Here's how the part is built. I have some questions about the finished solid (model axes, mm). A direction names the side the tool comes from. Give positions to 0.01 mm unless a question says otherwise; leave off trailing zeros. Loops run counter-clockwise (first coordinate to the right, second up) from the corner with the lowest first, then second, coordinate; pieces in that order, holes last. Notation, with made-up numbers: (67.5, 89.25) -> (123.5, 89.25) arc R27 ccw to (123.5, 106.25) -> close; hole circle Ø5 at (89, 24). An arc over 180 degrees is marked (long way). Answer in a Markdown table with one row per item. Add a question column.
Item 1: We'd pull the mould along Z, two halves only. Please class faces 1 (the face through (-3, 12.8, 2)), 2 (the face through (-9.24, 1.41, 3.52)): released by +Z, released by -Z, zero draft, split by the parting line, or undercut.
Item 2: If we section it at A-A (x = -12): Write out the boundary of the cut face in (y, z), then the cut area to 3 significant figures.
Item 3: If I drill on line 1 (X direction, y = 0.25, z = 0.5); line 2 (Y direction, x = -1, z = 2.5); line 3 (X direction, y = -8, z = 1.05), over which ranges is the centre line in solid material (lowest first)?
Item 4: For P1, Ø1, axis at x = -13.5, z = 4, coming from the +Y side; P2, Ø1, axis at x = 7, z = 1.5, coming from the -Y side, each with a flat end and sliding along its axis, tell me the tip position at first contact or that it passes through.
Item 5: If we section it at C-C (x = 9.5): Write out the boundary of the cut face in (y, z), then the cut area to 3 significant figures.
Item 6: If we section it at B-B (z = 4.2): Write out the boundary of the cut face in (x, y).
Item 7: Which directions (+Z, -Z, +X, -X, +Y, -Y) give clear straight access to the entire face, cutting with the end or side of a thin tool? Please do faces 3 (the face through (-9.24, -11.99, 2.46)), 4 (the face through (2.94, 1.35, 3.52)).
```python
from build123d import *

# Parameters (mm, degrees)
ESQUISSE1_W                       = 34
ESQUISSE1_H                       = 25.6
ESQUISSE1_R                       = 1.7
ESQUISSE1_R_2                     = 2.6
BOSS_EXTRU_1_DEPTH                = 5
ENL_V_MAT_EXTRU_2_DEPTH           = 3
ENL_V_MAT_EXTRU_2_DRAFT           = -5
ENL_V_MAT_EXTRU_2_PROFILE_2_DEPTH = 3
ENL_V_MAT_EXTRU_2_PROFILE_2_DRAFT = -5
ENL_V_MAT_EXTRU_3_DEPTH           = 10
CONG_1_R                          = 4


with BuildPart() as part:
    # Esquisse1 → Boss.-Extru.1 (new body)
    with BuildSketch(Plane.XY):
        with Locations((-3.241443597, 0)):
            Rectangle(ESQUISSE1_W, ESQUISSE1_H)
        with Locations((-11.726724972, 0)):
            Circle(ESQUISSE1_R, mode=Mode.SUBTRACT)
        with Locations((-3.241443597, 8.485281374)):
            Circle(ESQUISSE1_R_2, mode=Mode.SUBTRACT)
        with Locations(Location((-3.241443597, -8.485281374, 0), (0, 0, 180))):
            Circle(ESQUISSE1_R_2, mode=Mode.SUBTRACT)
        with Locations(Location((5.243837777, 0, 0), (0, 0, 180))):
            Circle(ESQUISSE1_R, mode=Mode.SUBTRACT)
    extrude(amount=BOSS_EXTRU_1_DEPTH)


with BuildPart() as enl_v_mat_extru_2_tool:
    # Esquisse3 → Enlèv. mat.-Extru.2 (with draft: the straight prism first)
    with BuildSketch(Plane.XY.offset(5)):
        Polygon((-8.278451106, 0), (-10.002588039, 2.986292767), (-13.450861905, 2.986292767), (-15.174998837, 0), (-13.450861905, -2.986292767), (-10.002588039, -2.986292767), align=None)
    extrude(amount=-ENL_V_MAT_EXTRU_2_DEPTH)
    # Enlèv. mat.-Extru.2: the draft: its side faces are tilted about the plane it starts from
    enl_v_mat_extru_2_sides = [enl_v_mat_extru_2_tool.faces().sort_by_distance(p)[0] for p in [
        (-9.140519572, 1.493146384, 3.5),
        (-11.726724972, 2.986292767, 3.5),
        (-14.312930371, 1.493146384, 3.5),
        (-14.312930371, -1.493146384, 3.5),
        (-11.726724972, -2.986292767, 3.5),
        (-9.140519572, -1.493146384, 3.5),
    ]]
    draft(enl_v_mat_extru_2_sides, Plane.XY.offset(5), ENL_V_MAT_EXTRU_2_DRAFT)


with BuildPart() as part_1:
    add(part.part)

    # Enlèv. mat.-Extru.2: cut by enl_v_mat_extru_2_tool
    add(enl_v_mat_extru_2_tool.part, mode=Mode.SUBTRACT)


with BuildPart() as enl_v_mat_extru_2_profile_2_tool:
    # Esquisse3 → Enlèv. mat.-Extru.2 profile 2 (with draft: the straight prism first)
    with BuildSketch(Plane.XY.offset(5)):
        Polygon((8.476999284, 0), (6.860418531, 2.8), (3.627257023, 2.8), (2.010676269, 0), (3.627257023, -2.8), (6.860418531, -2.8), align=None)
    extrude(amount=-ENL_V_MAT_EXTRU_2_PROFILE_2_DEPTH)
    # Enlèv. mat.-Extru.2 profile 2: the draft: its side faces are tilted about the plane it starts from
    enl_v_mat_extru_2_profile_2_sides = [enl_v_mat_extru_2_profile_2_tool.faces().sort_by_distance(p)[0] for p in [
        (7.668708907, 1.4, 3.5),
        (5.243837777, 2.8, 3.5),
        (2.818966646, 1.4, 3.5),
        (2.818966646, -1.4, 3.5),
        (5.243837777, -2.8, 3.5),
        (7.668708907, -1.4, 3.5),
    ]]
    draft(enl_v_mat_extru_2_profile_2_sides, Plane.XY.offset(5), ENL_V_MAT_EXTRU_2_PROFILE_2_DRAFT)


with BuildPart() as part_2:
    add(part_1.part)

    # Enlèv. mat.-Extru.2 profile 2: cut by enl_v_mat_extru_2_profile_2_tool
    add(enl_v_mat_extru_2_profile_2_tool.part, mode=Mode.SUBTRACT)

    # Esquisse4 → Enlèv. mat.-Extru.3 (cut)
    with BuildSketch(Plane(origin=(0, 0, 0), x_dir=(-1, 0, 0), z_dir=(0, 0, -1))):
        with BuildLine():
            Line((10.241443597, 12.8), (20.241443597, 12.8))
            Line((20.241443597, 12.8), (20.241443597, 2.8))
            ThreePointArc((20.241443597, 2.8), (13.170375785, 5.728932188), (10.241443597, 12.8))
        make_face()
        with BuildLine():
            Line((20.241443597, -12.8), (20.241443597, -2.8))
            ThreePointArc((20.241443597, -2.8), (13.170375785, -5.728932188), (10.241443597, -12.8))
            Line((10.241443597, -12.8), (20.241443597, -12.8))
        make_face()
        with BuildLine():
            Line((-3.758556403, -12.8), (-13.758556403, -12.8))
            Line((-13.758556403, -12.8), (-13.758556403, -2.8))
            ThreePointArc((-13.758556403, -2.8), (-6.687488591, -5.728932188), (-3.758556403, -12.8))
        make_face()
        with BuildLine():
            Line((-13.758556403, 12.8), (-13.758556403, 2.8))
            ThreePointArc((-13.758556403, 2.8), (-6.687488591, 5.728932188), (-3.758556403, 12.8))
            Line((-3.758556403, 12.8), (-13.758556403, 12.8))
        make_face()
    extrude(amount=-ENL_V_MAT_EXTRU_3_DEPTH, mode=Mode.SUBTRACT)

    # Congé1
    # the kernel refuses this fillet: 4 mm, written as the material it takes off along each edge
    with BuildSketch(Plane(origin=(-10.241443597, -12.8, -8.541019662), x_dir=(1, 0, 0), z_dir=(0, 0, 1)), Plane(origin=(-20.241443597, 2.8, -8.541019662), x_dir=(0, -1, 0), z_dir=(0, 0, 1)), Plane(origin=(3.758556403, 12.8, -8.541019662), x_dir=(-1, 0, 0), z_dir=(0, 0, 1))) as cong_1_piece_1:
        with BuildLine():
            CenterArc((3.416407865, 4), CONG_1_R, 196.601549599, 73.398450401)
            ThreePointArc((-0.416851525, 2.857142857), (-0.104761631, 1.443695821), (0, 0))
            Line((0, 0), (3.416407865, 0))
        make_face()
    extrude(amount=22.082039325, mode=Mode.SUBTRACT)
    with BuildSketch(Plane(origin=(-20.241443597, -2.8, -8.541019662), x_dir=(0.9895238368781002, -0.14436958214957515, 0), z_dir=(0, 0, 1)), Plane(origin=(-10.241443597, 12.8, -8.541019662), x_dir=(-0.14436958214957388, -0.9895238368781005, 0), z_dir=(0, 0, 1)), Plane(origin=(13.758556403, 2.8, -8.541019662), x_dir=(-0.9895238368781005, 0.14436958214957332, 0), z_dir=(0, 0, 1))) as cong_1_piece_2:
        with BuildLine():
            CenterArc((3.464869972, 3.958095348), CONG_1_R, 188.300774799, 73.398450401)
            Line((-0.493225376, 3.380617019), (0, 0))
            ThreePointArc((0, 0), (1.443695821, 0.104761631), (2.887391643, 0))
        make_face()
    extrude(amount=22.082039325, mode=Mode.SUBTRACT)
    with BuildSketch(Plane(origin=(3.758556403, -12.8, -8.541019662), x_dir=(-1, 0, 0), z_dir=(0, 0, 1))) as cong_1_piece_3:
        with BuildLine():
            CenterArc((3.416407865, -4), CONG_1_R, 90, 73.398450401)
            ThreePointArc((-0.416851525, -2.857142857), (-0.104761631, -1.443695821), (0, 0))
            Line((0, 0), (3.416407865, 0))
        make_face()
    extrude(amount=22.082039325, mode=Mode.SUBTRACT)
    with BuildSketch(Plane(origin=(13.758556403, -2.8, -8.541019662), x_dir=(-0.9895238368781001, -0.14436958214957546, 0), z_dir=(0, 0, 1))) as cong_1_piece_4:
        with BuildLine():
            CenterArc((3.464869972, -3.958095348), CONG_1_R, 98.3007748, 73.398450401)
            Line((-0.493225376, -3.380617019), (0, 0))
            ThreePointArc((0, 0), (1.443695821, -0.104761631), (2.887391643, 0))
        make_face()
    extrude(amount=22.082039325, mode=Mode.SUBTRACT)


solid = part_2.part
```
Recorded:
| question | item | result |
|---|---|---|
| 1 | face 1 | zero draft |
| 1 | face 2 | released by +Z |
| 2 | outline | (-7.14, 0) -> (-1.68, 0) -> (-1.68, 2) -> (-2.72, 2) -> (-2.99, 5) -> (-7.14, 5) -> close; (1.68, 0) -> (7.14, 0) -> (7.14, 5) -> (2.99, 5) -> (2.72, 2) -> (1.68, 2) -> close |
| 2 | area | 47.5 mm^2 |
| 3 | line 1 | x = -20.15 to -13.41, -10.05 to 3.56, 6.93 to 13.66 |
| 3 | line 2 | y = -12.8 to -9.8, -7.17 to 7.17, 9.8 to 12.8 |
| 3 | line 3 | x = -11.47 to -5.8, -0.69 to 4.99 |
| 4 | P1 | stops at y = 5.9 |
| 4 | P2 | stops at y = -5.92 |
| 5 | outline | (-3.75, 0) -> (3.75, 0) -> (3.75, 5) -> (-3.75, 5) -> close |
| 5 | area | 37.5 mm^2 |
| 6 | outline | (-20.19, 0) arc R4 ccw to (-17.38, -3.22) arc R10 cw to (-10.66, -9.94) arc R4 ccw to (-6.83, -12.8) -> (0.34, -12.8) arc R4 ccw to (4.18, -9.94) arc R10 cw to (10.9, -3.22) arc R4 ccw to (13.71, 0) arc R4 ccw to (10.9, 3.22) arc R10 cw to (4.18, 9.94) arc R4 ccw to (0.34, 12.8) -> (-6.83, 12.8) arc R4 ccw to (-10.66, 9.94) arc R10 cw to (-17.38, 3.22) arc R4 ccw to start; hole (-15.09, 0) -> (-13.41, -2.92) -> (-10.04, -2.92) -> (-8.36, 0) -> (-10.04, 2.92) -> (-13.41, 2.92) -> close; hole circle Ø5.2 at (-3.24, -8.49); hole circle Ø5.2 at (-3.24, 8.49); hole (2.09, 0) -> (3.67, -2.73) -> (6.82, -2.73) -> (8.4, 0) -> (6.82, 2.73) -> (3.67, 2.73) -> close |
| 7 | face 3 | +Z, -Z, -X, -Y |
| 7 | face 4 | +Z |
